Here's how the part is built. I have some questions about the finished solid (model axes, mm). Face numbers are marked on the shaded views. A direction names the side the tool comes from. Give positions to 0.01 mm unless a question says otherwise; leave off trailing zeros. Loops run counter-clockwise (first coordinate to the right, second up) from the corner with the lowest first, then second, coordinate; pieces in that order, holes last.
Q1. Thinking about a two-plate mould opening in Y: for the marked faces 1, 2 and 3, which applies, pulls with the +Y half, pulls with the -Y half, needs draft (parallel to the pull), parting line crosses it, or undercut?
Q2. Suppose I cut it at D-D (x = 4.75). List the corners of the cut face in (y, z) for me, and give its area (4 significant figures).
Q3. Suppose I cut it at B-B (y = -1.25). List the corners of the cut face in (x, z) for me.
Q4. Suppose I cut it at A-A (x = 18.75). List the corners of the cut face in (y, z) for me, and give its area (3 significant figures).
Q5. For the marked faces 4, 5, 6 and 7, which set-ups out of +Z, -Z, +X, -X, +Y, -Y let a thin tool reach every point of the face, with its end or its side?
Q6. Suppose I cut it at C-C (z = 8.5). List the corners of the cut face in (x, y) for me.
Q7. I need wall thicknesses on probe 1 along Y at (x, z) = (16.5, 11.25); probe 2 along Z at (x, y) = (20, 1.75); probe 3 along Z at (x, y) = (3.75, 2.5). Which ranges of each line are inside material? Lowest first, please.
Q8. I'm going to push flat-ended pins straight in: P1, Ø2, axis at x = 1.5, y = 3, coming from the -Z side; P2, Ø0.6, axis at x = 20.5, y = -2.5, coming from the +Z side; P3, Ø1.5, axis at x = 20, z = 4.5, coming from the -Y side. Where does each tip first touch, or does it pass through?
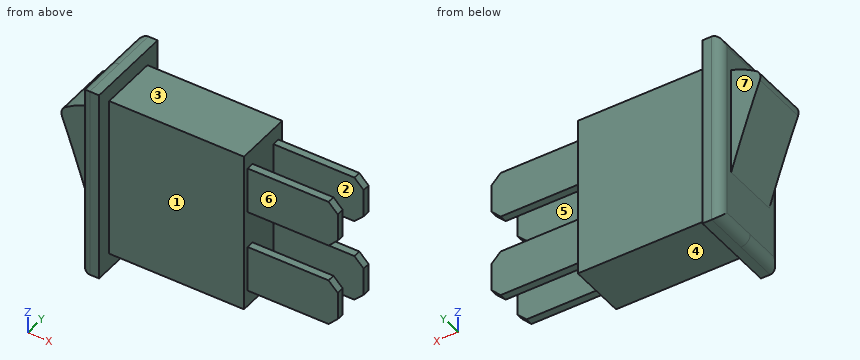
```python
from build123d import *

# Parameters (mm, degrees)
BOSS_EXTRU_1_DEPTH           = 3.1
ESQUISSE2_W                  = 2
ESQUISSE2_H                  = 21
BOSS_EXTRU_2_DEPTH           = 1.65
ESQUISSE3_W                  = 5
ESQUISSE3_H                  = 0.8
BOSS_EXTRU_3_DEPTH           = 9.7
CHANFREIN1_SIZE              = 1
CONG_1_R                     = 1
CHANFREIN1_OF_SYM_TRIE1_SIZE = 1
CONG_1_OF_SYM_TRIE1_R        = 1


with BuildPart() as part:
    # Esquisse1 → Boss.-Extru.1 (new body)
    with BuildSketch(Plane(origin=(0, 0, 0), x_dir=(1, 0, 0), z_dir=(0, 1, 0))):
        with BuildLine():
            Line((0, 0), (0, 1.75))
            Line((0, 1.75), (-2, 1.75))
            Line((-2, 1.75), (-2, -4.33188101))
            ThreePointArc((-2, -4.33188101), (-3.484320415, -8.968776107), (-5.089343046, -13.565286261))
            ThreePointArc((-5.089343046, -13.565286261), (-5.102407263, -14.21094477), (-4.718121663, -14.729953597))
            ThreePointArc((-4.718121663, -14.729953597), (-3.408583651, -15.498315478), (-2, -16.065026941))
            Line((-2, -16.065026941), (-2, -19.25))
            Line((-2, -19.25), (0, -19.25))
            Line((0, -19.25), (0, -17.5))
            Line((0, -17.5), (14.5, -17.5))
            Line((14.5, -17.5), (14.5, 0))
            Line((14.5, 0), (0, 0))
        make_face()
    boss_extru_1 = extrude(amount=BOSS_EXTRU_1_DEPTH)

    # Esquisse2 → Boss.-Extru.2 (add)
    with BuildSketch(Plane(origin=(0, 3.1, 0), x_dir=(1, 0, 0), z_dir=(0, 1, 0))):
        with Locations((-1, -8.75)):
            Rectangle(ESQUISSE2_W, ESQUISSE2_H)
    boss_extru_2 = extrude(amount=BOSS_EXTRU_2_DEPTH)

    # Esquisse3 → Boss.-Extru.3 (add)
    with BuildSketch(Plane(origin=(14.5, 0, 0), x_dir=(0, 0, -1), z_dir=(1, 0, 0))):
        with Locations((-13.25, 2.1)):
            Rectangle(ESQUISSE3_W, ESQUISSE3_H)
        with Locations((-4.25, 2.1)):
            Rectangle(ESQUISSE3_W, ESQUISSE3_H)
    boss_extru_3 = extrude(amount=BOSS_EXTRU_3_DEPTH)

    # Chanfrein1
    chanfrein1_edges = [part.edges().sort_by_distance(p)[0] for p in [
        (24.2, 2.1, 15.75),
        (24.2, 2.1, 10.75),
        (24.2, 2.1, 6.75),
        (24.2, 2.1, 1.75),
    ]]
    chamfer(chanfrein1_edges, length=CHANFREIN1_SIZE)

    # Congé1
    cong_1_edges = [part.edges().sort_by_distance(p)[0] for p in [
        (-2, 2.375, 19.25),
        (-2, 2.375, -1.75),
        (-2, 4.75, 8.75),
    ]]
    fillet(cong_1_edges, radius=CONG_1_R)

    # Symétrie1: Boss.-Extru.1, Boss.-Extru.2, Boss.-Extru.3 across plane
    add(boss_extru_1.mirror(Plane(origin=(1.115166408, 0, 6.288257404), x_dir=(0, 0, 1), z_dir=(0, 1, 0))))
    add(boss_extru_2.mirror(Plane(origin=(1.115166408, 0, 6.288257404), x_dir=(0, 0, 1), z_dir=(0, 1, 0))))
    add(boss_extru_3.mirror(Plane(origin=(1.115166408, 0, 6.288257404), x_dir=(0, 0, 1), z_dir=(0, 1, 0))))

    # Chanfrein1 of Symétrie1
    chanfrein1_of_sym_trie1_edges = [part.edges().sort_by_distance(p)[0] for p in [
        (24.2, -2.1, 15.75),
        (24.2, -2.1, 10.75),
        (24.2, -2.1, 6.75),
        (24.2, -2.1, 1.75),
    ]]
    chamfer(chanfrein1_of_sym_trie1_edges, length=CHANFREIN1_OF_SYM_TRIE1_SIZE)

    # Congé1 of Symétrie1
    cong_1_of_sym_trie1_edges = [part.edges().sort_by_distance(p)[0] for p in [
        (-2, -2.375, 19.25),
        (-2, -2.375, -1.75),
        (-2, -4.75, 8.75),
    ]]
    fillet(cong_1_of_sym_trie1_edges, radius=CONG_1_OF_SYM_TRIE1_R)


solid = part.part
```
Solutions:
1. face 1: pulls with the -Y half
1. face 2: undercut
1. face 3: needs draft
2. outline: (-3.1, 0) - (3.1, 0) - (3.1, 17.5) - (-3.1, 17.5) - close
2. area: 108.5 mm2
3. outline: (-5.09, 13.57) arc R186.24 cw to (-2, 4.33) - (-2, -0.75) arc R1 ccw to (-1, -1.75) - (0, -1.75) - (0, 0) - (14.5, 0) - (14.5, 17.5) - (0, 17.5) - (0, 19.25) - (-1, 19.25) arc R1 ccw to (-2, 18.25) - (-2, 16.07) arc R10.26 ccw to (-4.72, 14.73) arc R1 ccw to start
4. outline: (-2.5, 1.75) - (-1.7, 1.75) - (-1.7, 6.75) - (-2.5, 6.75) - close; (-2.5, 10.75) - (-1.7, 10.75) - (-1.7, 15.75) - (-2.5, 15.75) - close; (1.7, 1.75) - (2.5, 1.75) - (2.5, 6.75) - (1.7, 6.75) - close; (1.7, 10.75) - (2.5, 10.75) - (2.5, 15.75) - (1.7, 15.75) - close
4. area: 16.0 mm2
5. face 4: -Z, +X, +Y, -Y
5. face 5: +Z, -Z, +X
5. face 6: +Z, -Z, +X, -Y
5. face 7: +Z, -Z, -X, +Y
6. outline: (-3.33, -3.1) - (-2, -3.1) - (-2, -3.75) arc R1 ccw to (-1, -4.75) - (0, -4.75) - (0, -3.1) - (14.5, -3.1) - (14.5, 3.1) - (0, 3.1) - (0, 4.75) - (-1, 4.75) arc R1 ccw to (-2, 3.75) - (-2, 3.1) - (-3.33, 3.1) - close
7. probe 1: y = -2.5 to -1.7, 1.7 to 2.5
7. probe 2: z = 1.75 to 6.75, 10.75 to 15.75
7. probe 3: z = 0 to 17.5
8. P1: stops at z = 0
8. P2: stops at z = 15.75
8. P3: stops at y = -2.5
